Input: dimensioned drawing with shaded views. Units: mm. Origin: part minimum x, y, z. Coordinates: 2 decimals unless noted, no trailing zeros. Loops run counter-clockwise (first coordinate to the right, second up) from the corner with the lowest first, then second, coordinate; pieces in that order, holes last.
Item 1: Section B-B on z = 1.5. Return loops of the section in (x, y) (1 decimal).
Item 2: Ray query, line 1 along Y through (x, z) = (64.5, 4.75); line 2 along Y through (x, z) = (42.5, 3.25); line 3 along X through (y, z) = (64.5, 3.75) (1 decimal). Return the intervals inside material, ascending.
Item 3: Section A-A on y = 61. Return loops of the section in (x, z) (1 decimal), and give its area (3 significant figures).
Item 4: Section C-C on x = 62.5. Return loops of the section in (y, z), and give its area (3 significant figures).
Item 5: Section D-D on x = 12.5. Return loops of the section in (y, z).
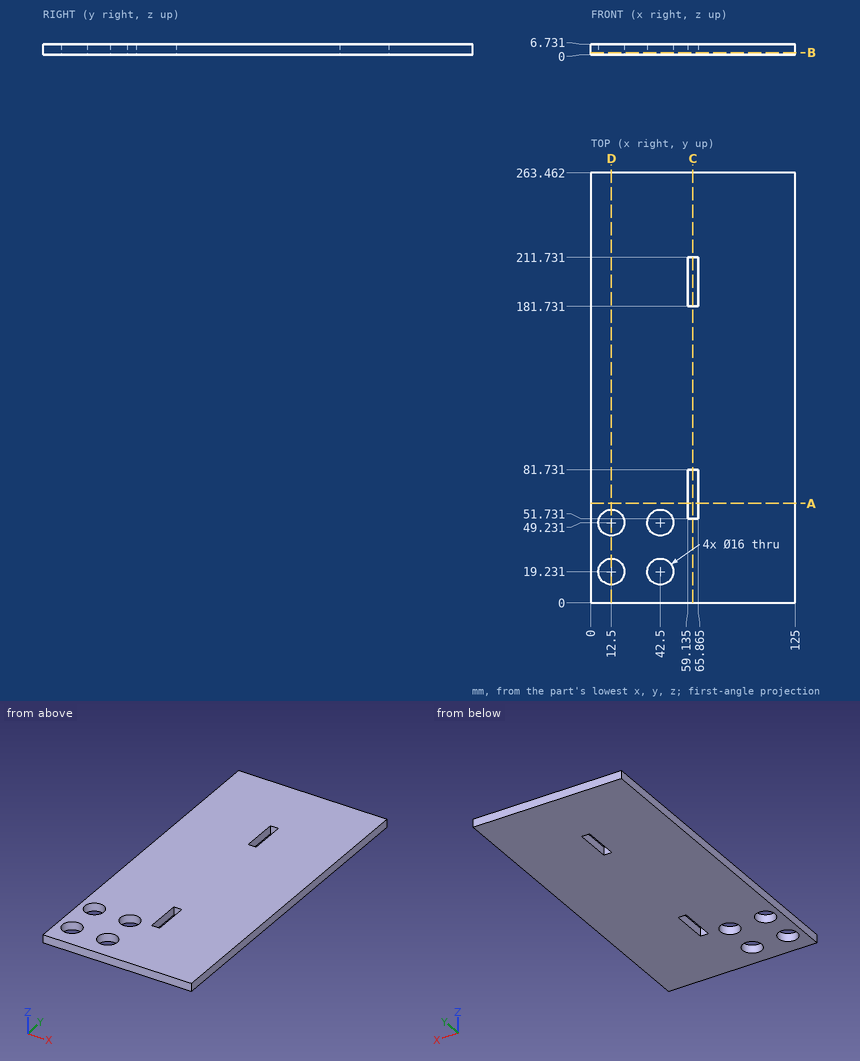
Results found:
1. outline: (0, 0) - (125, 0) - (125, 263.5) - (0, 263.5) - close; hole circle Ø16 at (12.5, 19.2); hole circle Ø16 at (12.5, 49.2); hole circle Ø16 at (42.5, 19.2); hole circle Ø16 at (42.5, 49.2); hole (59.1, 51.7) - (65.9, 51.7) - (65.9, 81.7) - (59.1, 81.7) - close; hole (59.1, 181.7) - (65.9, 181.7) - (65.9, 211.7) - (59.1, 211.7) - close
2. line 1: y = 0 to 51.73, 81.73 to 181.73, 211.73 to 263.46
2. line 2: y = 0 to 11.23, 27.23 to 41.23, 57.23 to 263.46
2. line 3: x = 0 to 59.1, 65.9 to 125
3. outline: (0, 0) - (59.1, 0) - (59.1, 6.7) - (0, 6.7) - close; (65.9, 0) - (125, 0) - (125, 6.7) - (65.9, 6.7) - close
3. area: 796 mm2
4. outline: (0, 0) - (51.73, 0) - (51.73, 6.73) - (0, 6.73) - close; (81.73, 0) - (181.73, 0) - (181.73, 6.73) - (81.73, 6.73) - close; (211.73, 0) - (263.46, 0) - (263.46, 6.73) - (211.73, 6.73) - close
4. area: 1,370 mm2
5. outline: (0, 0) - (11.23, 0) - (11.23, 6.73) - (0, 6.73) - close; (27.23, 0) - (41.23, 0) - (41.23, 6.73) - (27.23, 6.73) - close; (57.23, 0) - (263.46, 0) - (263.46, 6.73) - (57.23, 6.73) - close
